from build123d import *

# Parameters (mm, degrees)
SKETCH1_R                = 77.321
SKETCH1_R_2              = 39.6875
BOSS_EXTRUDE1_DEPTH      = 15
SKETCH2_R                = 87.321
SKETCH2_R_2              = 77.321
BOSS_EXTRUDE2_DEPTH      = 40
BOSS_EXTRUDE2_DEPTH_BACK = 15
BOSS_EXTRUDE3_DEPTH      = 40
SKETCH4_R                = 2.5
CUT_EXTRUDE1_DEPTH       = 21.359049754
CIRPATTERN1_COUNT        = 6


with BuildPart() as part:
    # Sketch1 → Boss-Extrude1 (new body)
    with BuildSketch(Plane(origin=(0, 0, 0), x_dir=(1, 0, 0), z_dir=(0, 1, 0))):
        Circle(SKETCH1_R)
        Circle(SKETCH1_R_2, mode=Mode.SUBTRACT)
    extrude(amount=BOSS_EXTRUDE1_DEPTH)

    # Sketch2 → Boss-Extrude2 (add, two sides)
    with BuildSketch(Plane(origin=(0, 15, 0), x_dir=(1, 0, 0), z_dir=(0, 1, 0))) as boss_extrude2_sk:
        Circle(SKETCH2_R)
        Circle(SKETCH2_R_2, mode=Mode.SUBTRACT)
    extrude(amount=BOSS_EXTRUDE2_DEPTH)
    extrude(boss_extrude2_sk.sketch, amount=-BOSS_EXTRUDE2_DEPTH_BACK)

    # Sketch3 → Boss-Extrude3 (add)
    with BuildSketch(Plane(origin=(0, 15, 0), x_dir=(1, 0, 0), z_dir=(0, 1, 0))):
        with BuildLine():
            ThreePointArc((-77.321, 0), (-66.961950246, -38.6605), (-38.6605, -66.961950246))
            Line((-38.6605, -66.961950246), (-77.321, 0))
        make_face()
        with BuildLine():
            Line((-77.321, 0), (-38.6605, 66.961950246))
            ThreePointArc((-38.6605, 66.961950246), (-66.961950246, 38.6605), (-77.321, 0))
        make_face()
        with BuildLine():
            Line((-38.6605, 66.961950246), (38.6605, 66.961950246))
            ThreePointArc((38.6605, 66.961950246), (0, 77.321), (-38.6605, 66.961950246))
        make_face()
        with BuildLine():
            Line((38.6605, 66.961950246), (77.321, 0))
            ThreePointArc((77.321, 0), (66.961950246, 38.6605), (38.6605, 66.961950246))
        make_face()
        with BuildLine():
            ThreePointArc((38.6605, -66.961950246), (66.961950246, -38.6605), (77.321, 0))
            Line((77.321, 0), (38.6605, -66.961950246))
        make_face()
        with BuildLine():
            ThreePointArc((-38.6605, -66.961950246), (0, -77.321), (38.6605, -66.961950246))
            Line((38.6605, -66.961950246), (-38.6605, -66.961950246))
        make_face()
    extrude(amount=BOSS_EXTRUDE3_DEPTH)

    # Sketch4 → Cut-Extrude1 (cut, through all)
    with BuildSketch(Plane.XY.offset(-66.961950246)):
        with Locations((0, 35)):
            Circle(SKETCH4_R)
    cut_extrude1 = extrude(amount=-CUT_EXTRUDE1_DEPTH, mode=Mode.SUBTRACT)

    # CirPattern1: Cut-Extrude1 ×6 about axis
    cirpattern1_axis = Axis((0, -246.98108496, 0), (0, 1, 0))
    for i in range(1, CIRPATTERN1_COUNT):
        add(cut_extrude1.rotate(cirpattern1_axis, i * 360 / CIRPATTERN1_COUNT), mode=Mode.SUBTRACT)


solid = part.part
The listing builds one solid part. Answer for the finished solid, in the listing's coordinates (mm). A direction names the side the tool comes from. Round coordinates to 2 decimals unless told otherwise and drop trailing zeros. Write each loop counter-clockwise with the first axis right and the second up, starting at its lowest first coordinate (ties: lowest second). Pieces come first, ordered by that corner, then holes. Notation, with made-up numbers: (79, 41) - (128, 41) arc R28 cw to (128, 63) - close; hole circle Ø9 at (15, 10.5). An arc over 180 degrees is marked (long way). Use one line per item in the form item = value. Start each with the question number.
Item 1: A cutting plane is placed at A-A (x = 0). Write down the section's boundary in (y, z), plus the area to 3 significant figures.
Item 2: A tool of negligible diameter and unlimited length cuts with its end or side. For faces 5 (the flat face through (-1, 30, -66.962)), 6 (the cylindrical face through (-0.54, 32.56, -77)), from which of +Z, -Z, +X, -X, +Y, -Y can it reach the whole face along a straight path? Write none if from no direction.
Item 3: Flat-ended cylindrical pins translate along their axes: pin 1 Ø6 at (y, z) = (46, 36) entering from -X; pin 2 Ø1.5 at (x, y) = (0.5, 19.5) entering from +Z; pin 3 Ø1 at (y, z) = (32.5, -53.5) entering from +X; pin 4 Ø8 at (x, z) = (-49, -49) entering from +Y. Find the tip coordinate at first contact, or state that the pin passes through.
Item 4: Find the intervals of material crossed by line 1 (Y direction, x = 0, z = 72.25); line 2 (Z direction, x = 1, y = 3); line 3 (X direction, y = 6, z = 0), in increasing order. Write a range as [from, to].
Item 5: A cutting plane is placed at C-C (z = -22). Write down the section's boundary in (x, y).
Item 6: A cutting plane is placed at B-B (y = 25). Write down the section's boundary in (x, z), plus the area to 3 significant figures.
Item 7: Determine the mould class of faces 1 (the cylindrical face through (0.54, 32.56, 77)), 2 (the flat face through (18, 0, 38)), 3 (the flat face through (58.261, 30.276, 33.012)), 4 (the cylindrical face through (-11.367, 27.885, -86.578)) for opening direction X: +X half, -X half, draft (parallel to the pull), parting line (faces both ways), or undercut.
Item 8: A cutting plane is placed at D-D (x = -28). Write down the section's boundary in (y, z), plus the area to 3 significant figures.
The answers:
q1.outline = (0, -87.32) - (32.5, -87.32) - (32.5, -66.96) - (15, -66.96) - (15, -39.69) - (0, -39.69) - close; (0, 39.69) - (15, 39.69) - (15, 66.96) - (32.5, 66.96) - (32.5, 87.32) - (0, 87.32) - close; (37.5, -87.32) - (55, -87.32) - (55, -66.96) - (37.5, -66.96) - close; (37.5, 66.96) - (55, 66.96) - (55, 87.32) - (37.5, 87.32) - close
q1.area = 2,850 mm^2
q2.face_5 = +Y
q2.face_6 = +Z, -Z
q3.pin_1 = -80.85
q3.pin_2 = 87.32
q3.pin_3 = 69.4
q3.pin_4 = 55
q4.line_1 = [0, 32.5], [37.5, 55]
q4.line_2 = [-87.32, -39.67], [39.67, 87.32]
q4.line_3 = [-87.32, -39.69], [39.69, 87.32]
q5.outline = (-84.5, 0) - (-33.03, 0) - (-33.03, 15) - (-64.62, 15) - (-64.62, 55) - (-84.5, 55) - close; (33.03, 0) - (84.5, 0) - (84.5, 55) - (64.62, 55) - (64.62, 15) - (33.03, 15) - close
q6.outline = circle Ø174.64 at (0, 0); hole (-77.32, 0) - (-38.66, -66.96) - (38.66, -66.96) - (77.32, 0) - (38.66, 66.96) - (-38.66, 66.96) - close
q6.area = 8,420 mm^2
q7.face_1 = undercut
q7.face_2 = draft
q7.face_3 = undercut
q7.face_4 = parting line
q8.outline = (0, -82.71) - (55, -82.71) - (55, -66.96) - (15, -66.96) - (15, -28.13) - (0, -28.13) - close; (0, 28.13) - (15, 28.13) - (15, 66.96) - (55, 66.96) - (55, 82.71) - (0, 82.71) - close
q8.area = 2,900 mm^2
